Geometry: final body of the model. Coordinates: model frame, mm. Face numbers are marked on the shaded views. A direction names the side the tool comes from. Give positions to 0.01 mm unless a question says otherwise; leave off trailing zeros. Write each loop counter-clockwise with the first axis right and the second up, starting at its lowest first coordinate (ties: lowest second). Pieces come first, ordered by that corner, then holes.
Autodesk Inventor part; units mm, degrees
ref_plane "YZ Plane" through (0, 0, 0) normal (1, 0, 0) x (0, 1, 0)
ref_plane "XZ Plane" through (0, 0, 0) normal (0, 1, 0) x (-1, 0, 0)
ref_plane "XY Plane" through (0, 0, 0) normal (0, 0, 1) x (1, 0, 0)
sketch "Sketch1" plane through (0, 0, 0) normal (0, 1, 0) x (-1, 0, 0)
  line L0 (76.2, 0) -> (76.2, -254)
  line L1 (76.2, -254) -> (0, -254)
  line L2 (0, -254) -> (0, 0)
  arc A0 (76.2, 0) -> (0, 0) centre (38.1, 0) ccw
extrude "Extrusion1" add sketch "Sketch1" along normal blind 76.2
sketch "Sketch2" plane through (0, 0, 0) normal (1, 0, 0) x (0, 0, -1)
  line L0 (-38.1, 25.4) -> (25.4, 25.4)
  line L1 (25.4, 25.4) -> (25.4, 50.8)
  line L2 (25.4, 50.8) -> (-38.1, 50.8)
  line L3 (-38.1, 0) -> (-38.1, 76.2)
  line L4 (-38.1, 38.1) -> (25.4, 50.8) construction
  line L5 (25.4, 25.4) -> (-38.1, 38.1) construction
  line L6 (-38.1, 50.8) -> (-38.1, 25.4)
  point P0 (0, 0)
extrude "Extrusion2" cut sketch "Sketch2" against normal blind 111.125
sketch "Sketch3" plane through (0, 76.2, 0) normal (0, 1, 0) x (1, 0, 0)
  point P0 (0, 0)
  point P1 (-39.0791, -13.8463)
hole "Hole1" at (-39.0791, 76.2, 13.8463) direction (0, -1, 0) diameter 12.7 depth 98.425 tip angle 118
sketch "Sketch5" plane through (0, 0, -254) normal (0, 0, -1) x (-1, 0, 0)
  line L0 (76.2, 0) -> (0, 0)
  line L1 (51.7791, 76.2) -> (51.7791, 0)
  line L2 (51.7791, 0) -> (26.3791, 0)
  line L3 (26.3791, 0) -> (26.3791, 76.2)
  line L4 (32.7291, 76.2) -> (45.4291, 76.2)
  line L5 (76.2, 76.2) -> (0, 76.2)
  line L6 (51.7791, 76.2) -> (24.7587, 76.2)
  point P0 (39.0791, 76.2)
extrude "Extrusion3" cut sketch "Sketch5" against normal blind 63.5
sketch "Sketch6" plane through (0, 0, 0) normal (1, 0, 0) x (0, 0, -1)
  point P0 (0, 0)
  point P1 (230.7386, 44.6045)
hole "Hole2" at (0, 44.6045, -230.7386) direction (-1, 0, 0) diameter 12.7 depth 98.425 tip angle 118
properties part number "SecondChain"
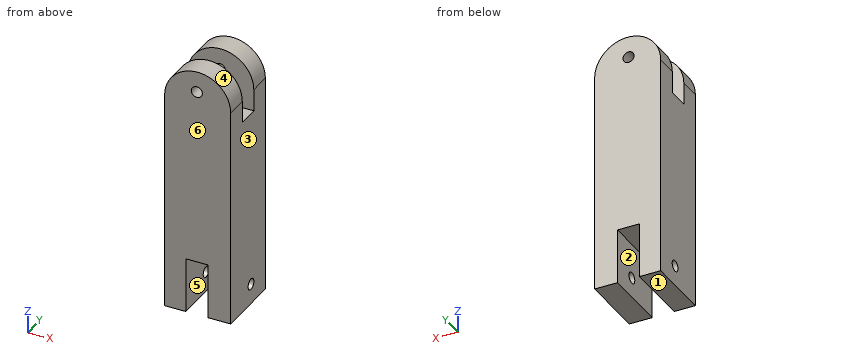
Q1. Section A-A on y = 34. Output: boundary loops of the cut face in (x, z).
Filled sheet:
outline: (-76.2, -254) - (-51.78, -254) - (-51.78, -190.5) - (-26.38, -190.5) - (-26.38, -254) - (0, -254) - (0, -25.4) - (-76.2, -25.4) - close
Q2. Pull-direction query (X, two-part tool) for the marked faces 1, 2, 3 and 4; classes: released by +X, released by -X, zero draft, split by the parting line, or undercut.
Filled sheet:
face 1: zero draft
face 2: undercut
face 3: released by +X
face 4: split by the parting line
Q3. Pin query (flat end, axial travel): P1, Ø20.5, axis at x = -40, y = 38, coming from the -Z side; P2, Ø6, axis at y = 24.5, z = 5, coming from the +X side; P3, Ø3, axis at y = 58, z = 2, coming from the +X side. Return the tip coordinate at first contact, or that it passes through.
Filled sheet:
P1: stops at z = -190.5
P2: stops at x = -0.05
P3: stops at x = 0
Q4. Section B-B on x = -59.5. Output: boundary loops of the cut face in (y, z).
Filled sheet:
outline: (0, -254) - (76.2, -254) - (76.2, 31.52) - (50.8, 31.52) - (50.8, -25.4) - (25.4, -25.4) - (25.4, 31.52) - (0, 31.52) - close; hole circle Ø12.7 at (44.6, -230.74)
Q5. Section C-C on y = 65.5. Output: boundary loops of the cut face in (x, z).
Filled sheet:
outline: (-76.2, -254) - (-51.78, -254) - (-51.78, -190.5) - (-26.38, -190.5) - (-26.38, -254) - (0, -254) - (0, 0) arc R38.1 ccw to (-76.2, 0) - close; hole circle Ø12.7 at (-39.08, 13.85)
Q6. Ray query, line 1 along X through (y, z) = (18.5, -212.5); line 2 along Z through (x, y) = (-38.5, 64); line 3 along Z through (x, y) = (-33.5, 17). Return the intervals inside material, ascending.
Filled sheet:
line 1: x = -76.2 to -51.78, -26.38 to 0
line 2: z = -190.5 to 7.52, 20.17 to 38.1
line 3: z = -190.5 to 10.81, 16.88 to 37.82
Q7. Access query for the marked faces 5 and 6. Directions: +Z, -Z, +X, -X, +Y, -Y. A direction counts if a zero-diameter tool reaches every point of the face in a straight line with its end or side. Return the directions, or none.
Filled sheet:
face 5: -Z, +Y, -Y
face 6: +Z, -Z, +X, -X, -Y
